Could you check a few things on this drawing? It's one solid part, dimensions in mm from its lowest x, y, z. A direction names the side the tool comes from. Round coordinates to 2 decimals unless told otherwise and drop trailing zeros. Order: outer loops, then holes, each group sorted by start corner. A loop starts at its lowest first (then second) coordinate and runs counter-clockwise, first axis right, second up. Notation, with made-up numbers: (-26.75, -24.75) - (31.25, -24.75) arc R21 ccw to (31.25, 9.25) - close; hole circle Ø6 at (50, 66.5). An arc over 180 degrees is marked (long way). Use one line per item in the form item = value.
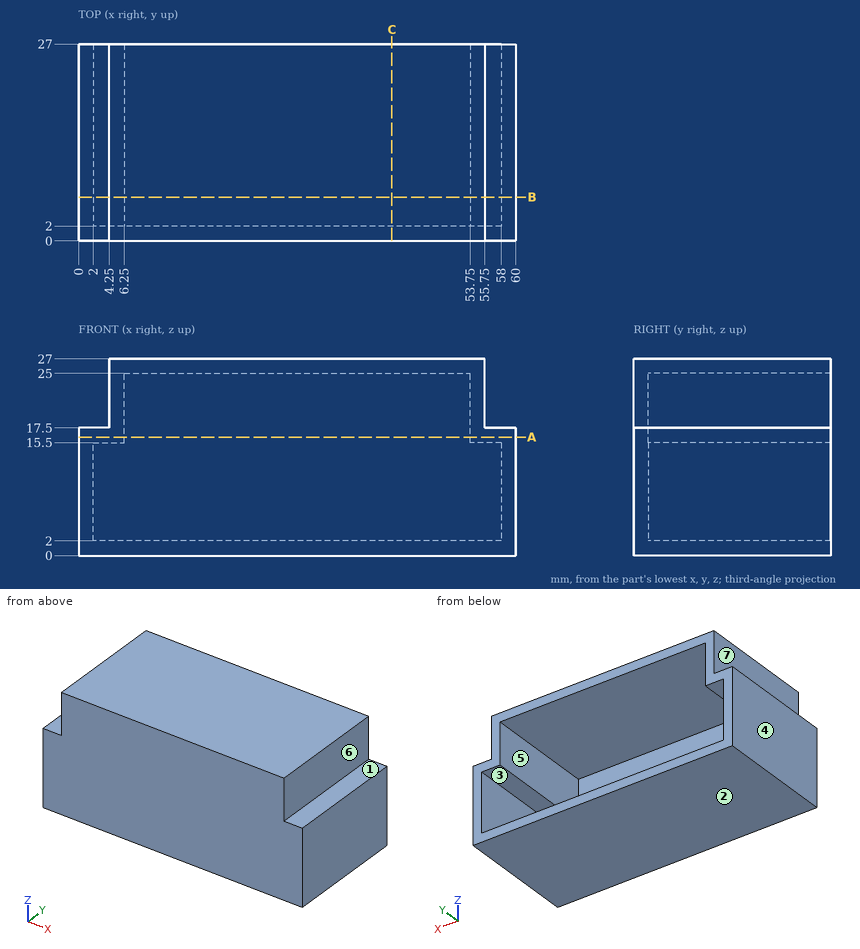
Item 1: If we mould it in two halves opening along Z, with no side actions, what happens to the marked faces 1, 2, 3 and 4? For each: released by +Z, released by -Z, zero draft, split by the parting line, or undercut.
Found:
face_1 = released by +Z
face_2 = released by -Z
face_3 = undercut
face_4 = zero draft
Item 2: Imagine slicing it at B-B on y = 6. Please give me the cut outline in (x, z), plus the area to 3 significant figures.
Found:
outline = (0, 0) - (60, 0) - (60, 17.5) - (55.75, 17.5) - (55.75, 27) - (4.25, 27) - (4.25, 17.5) - (0, 17.5) - close; hole (2, 2) - (58, 2) - (58, 15.5) - (53.75, 15.5) - (53.75, 25) - (6.25, 25) - (6.25, 15.5) - (2, 15.5) - close
area = 332 mm2
Item 3: Will these pins go through, and if not, where does the flat tip stop? P1, Ø4, axis at y = 12.5, z = 13.5, coming from the -X side; P2, Ø3, axis at y = 11, z = 19.5, coming from the +X side; P3, Ø1.3, axis at x = 57, y = 18.5, coming from the +Z side; P4, Ø10.5, axis at y = 8, z = 24.5, coming from the -X side.
Found:
P1 = 0
P2 = 55.75
P3 = 17.5
P4 = 4.25
Item 4: For the marked faces 5, 6 and 7, which set-ups out of +Z, -Z, +X, -X, +Y, -Y let a thin tool reach every point of the face, with its end or its side?
Found:
face_5 = +Y
face_6 = +Z, +X, +Y, -Y
face_7 = +Z, -X, +Y, -Y
Item 5: I need wall thicknesses on L1, parallel to Z at x = 45.5, y = 15; L2, parallel to X at y = 23.25, z = 6.5; L3, parallel to X at y = 11.5, z = 19.25. Which ranges of each line are inside material? Lowest first, please.
Found:
L1 = 0 to 2, 25 to 27
L2 = 0 to 2, 58 to 60
L3 = 4.25 to 6.25, 53.75 to 55.75
Item 6: Imagine slicing it at C-C on x = 43. Please give me the cut outline in (y, z), plus the area to 3 significant figures.
Found:
outline = (0, 0) - (27, 0) - (27, 2) - (2, 2) - (2, 25) - (27, 25) - (27, 27) - (0, 27) - close
area = 154 mm2
Item 7: Imagine slicing it at A-A on z = 16.25. Please give me the cut outline in (x, y).
Found:
outline = (0, 0) - (60, 0) - (60, 27) - (53.75, 27) - (53.75, 2) - (6.25, 2) - (6.25, 27) - (0, 27) - close
